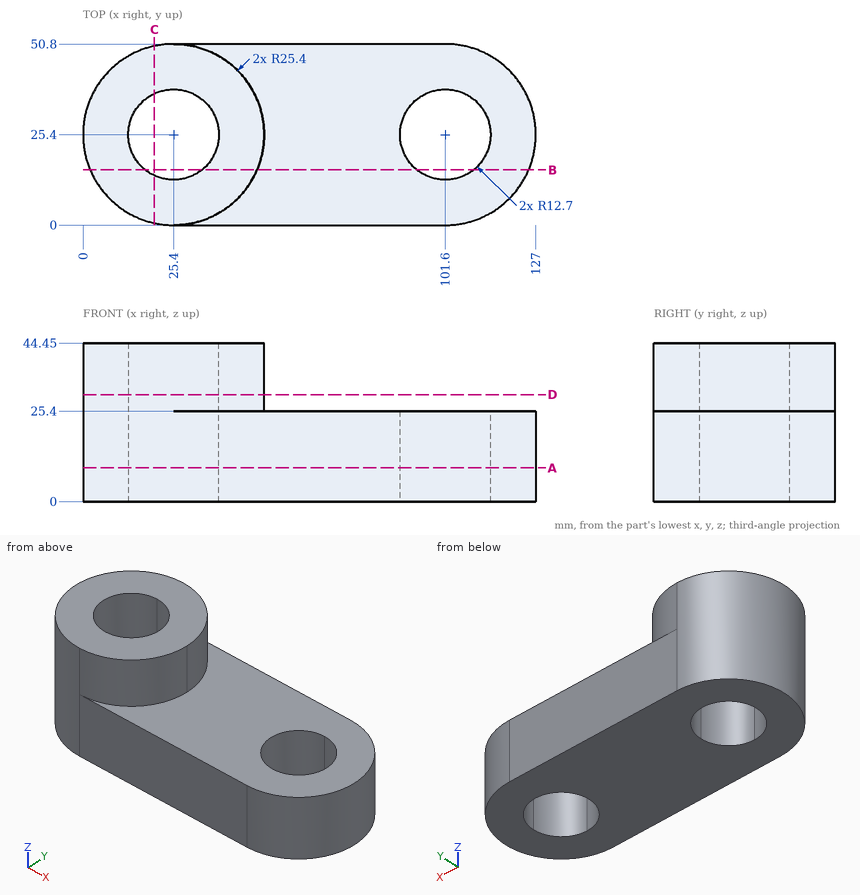
Study the drawing (mm; zero at the part's minimum x, y, z) and answer. Round coordinates to 2 decimals unless told otherwise and drop trailing zeros. Order: outer loops, then holes, each group sorted by start corner. A loop starts at its lowest first (then second) coordinate and runs counter-clockwise, first axis right, second up. Notation, with made-up numbers: (-22.5, -22) -> (-8.5, -22) arc R28 cw to (-8.5, 3) -> close; hole circle Ø9 at (24, 73.25). An arc over 180 degrees is marked (long way). Write each question's results on one line, items separated by ' | '. Start each with the question number.
Q1. Straight lines are drawn through the part: probe 1 along Y at (x, z) = (25, 3); probe 2 along X at (y, z) = (35.5, 15); probe 3 along Z at (x, y) = (119, 24). For each, find the intervals that lie inside material, in ascending order. Write a range as from..to.
Q2. Find section B-B (y = 15.5). Determine the outline of the cut face in (x, z).
Q3. Find section A-A (z = 9.5). Determine the outline of the cut face in (x, y), then the cut area to 3 significant figures.
Q4. Each of these flat-tipped pins is pushed along its axis until it touches: pin 1 (4 mm diameter, centred on x = 41, z = 31.5, fed in from -Y); pin 2 (5 mm diameter, centred on x = 90.5, y = 17.5, fed in from +Z); pin 3 (2 mm diameter, centred on y = 13, z = 5, fed in from +X). Where does it stop, or does it pass through?
Q5. Find section D-D (z = 30). Determine the outline of the cut face in (x, y).
Q6. Find section C-C (x = 20). Determine the outline of the cut face in (y, z), then the cut area to 3 significant figures.
Worked answers:
1) probe 1: y = 0..12.71, 38.09..50.8 | probe 2: x = 2.09..17.7, 33.1..93.9, 109.3..124.91 | probe 3: z = 0..25.4
2) outline: (2.01, 0) -> (17.45, 0) -> (17.45, 44.45) -> (2.01, 44.45) -> close; (33.35, 0) -> (93.65, 0) -> (93.65, 25.4) -> (48.79, 25.4) -> (48.79, 44.45) -> (33.35, 44.45) -> close; (109.55, 0) -> (124.99, 0) -> (124.99, 25.4) -> (109.55, 25.4) -> close
3) outline: (25.4, 0) -> (101.6, 0) arc R25.4 ccw to (101.6, 50.8) -> (25.4, 50.8) arc R25.4 ccw to start; hole circle Ø25.4 at (25.4, 25.4); hole circle Ø25.4 at (101.6, 25.4) | area: 4,880 mm2
4) pin 1: stops at y = 3.95 | pin 2: stops at z = 25.4 | pin 3: stops at x = 124.3
5) outline: (25.4, 0) arc R25.4 ccw to (50.8, 25.4) arc R25.4 ccw (long way) to start; hole circle Ø25.4 at (25.4, 25.4)
6) outline: (0.58, 0) -> (13.91, 0) -> (13.91, 44.45) -> (0.58, 44.45) -> close; (36.89, 0) -> (50.22, 0) -> (50.22, 44.45) -> (36.89, 44.45) -> close | area: 1,180 mm2
